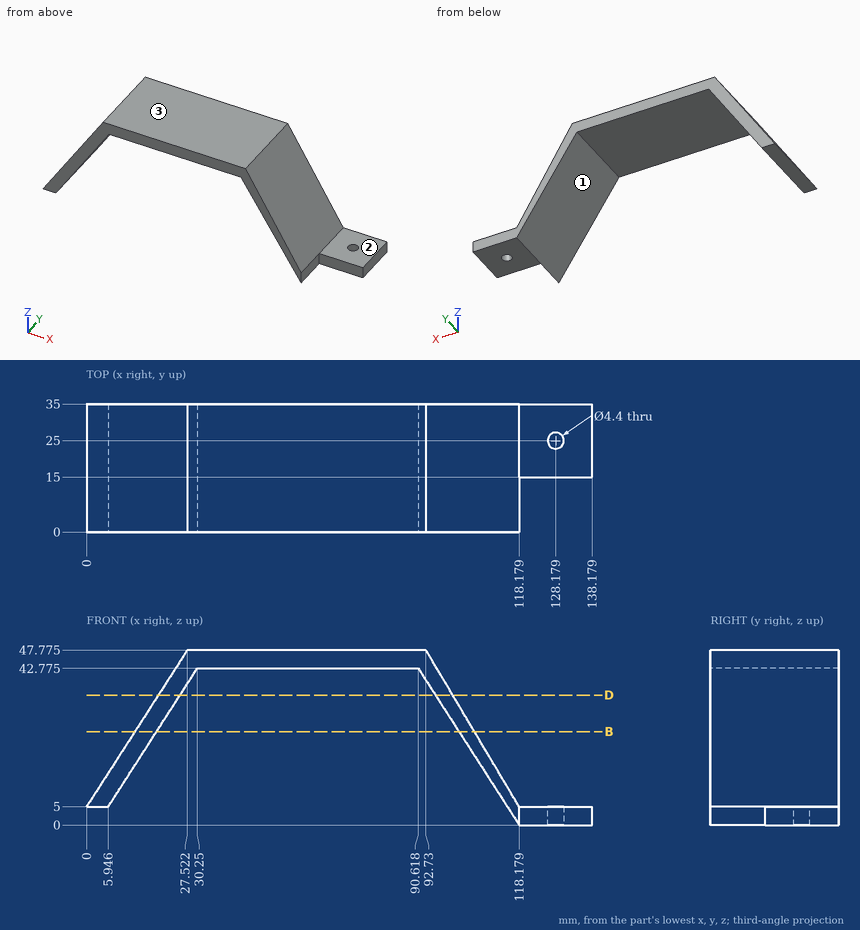
Geometry: see drawing. Coordinates: mm, zero at the bounding-box minimum. A direction names the side the tool comes from. Coordinates: 2 decimals unless noted, no trailing zeros. Loops run counter-clockwise (first coordinate to the right, second up) from the corner with the lowest first, then second, coordinate; pieces in that order, holes last.
(1) Section D-D on z = 35.5. Return the cut outline in (x, y) (1 decimal).
(2) Set-up query: the marked faces 1, 2 and 3. Return all of +Z, -Z, +X, -X, +Y, -Y with unobstructed straight access to the full face (end or side cutting, diameter ignored); none if empty.
(3) First-contact query: pin 1 Ø5 at (x, z) = (20.5, 41) entering from -Y; pin 2 Ø2.5 at (x, z) = (130.5, 2) entering from -Y; pin 3 Ø5 at (x, y) = (4, 21) entering from -Z; pin 4 Ø10 at (x, y) = (130.5, 26) entering from +Z. Flat tips, straight axial feed; report the tip coordinate or a pass-through.
(4) Material intervals for probe 1 along Z at (x, y) = (127, 22); probe 2 along Z at (x, y) = (48, 4) (1 decimal); probe 3 along X at (y, z) = (23, 38) (1 decimal), sorted ascending.
(5) Section B-B on z = 25.5. Return the cut outline in (x, y) (1 decimal).
Data:
1. outline: (19.6, 0) - (25.6, 0) - (25.6, 35) - (19.6, 35) - close; (95.3, 0) - (100, 0) - (100, 35) - (95.3, 35) - close
2. face 1: -Z, +Y, -Y
2. face 2: +Z, +X, +Y, -Y
2. face 3: +Z, +X, -X, +Y, -Y
3. pin 1: stops at y = 0
3. pin 2: stops at y = 15
3. pin 3: stops at z = 5
3. pin 4: stops at z = 5
4. probe 1: z = 0 to 5
4. probe 2: z = 42.8 to 47.8
4. probe 3: x = 21.2 to 27.2, 93.7 to 98.5
5. outline: (13.2, 0) - (19.1, 0) - (19.1, 35) - (13.2, 35) - close; (101.7, 0) - (106, 0) - (106, 35) - (101.7, 35) - close
